The listing builds one solid part. Answer for the finished solid, in the listing's coordinates (mm). A direction names the side the tool comes from. Give positions to 0.01 mm unless a question says otherwise; leave off trailing zeros. Write each loop counter-clockwise with the first axis right and the second up, starting at its lowest first coordinate (ties: lowest second). Pieces come first, ordered by that corner, then holes. Notation, with made-up numbers: (-3.5, -10) - (6.5, -10) arc R25 ccw to (6.5, 19) - close; hole circle Ø5 at (65.5, -8). An arc over 180 degrees is marked (long way). One line per question, with ' | ' between items. Start each with the question number.
1. Find the intervals of material crossed by L1, parallel to Z at x = 0, y = -12; L2, parallel to Z at x = 8, y = 29.5; L3, parallel to X at y = -1, z = 33, in increasing order. Write a range as from..to.
2. The mould has two halves that part along Z. Classify faces 1 (the face through (24.77, -0.89, -58.47)), 2 (the face through (-1, -63.5, 1)), 3 (the face through (-59.728, -0.889, -21.558)), 4 (the face through (69.85, -0.89, -0.14)): +Z half, -Z half, draft (parallel to the pull), parting line (faces both ways), or undercut.
3. Given P1, Ø5, axis at y = 37.5, z = 25.5, coming from the -X side; P2, Ø2, axis at y = 20, z = -40, coming from the -X side; P3, Ø8, axis at x = -8.5, z = -7, coming from the +Y side, each flat-ended and moving along its own axis, determine where each tip first touches the part or whether it passes through.
4. A cutting plane is placed at A-A (y = -33). Determine the outline of the cut face in (x, z), then the cut area to 3 significant figures.
5. For faces 5 (the face through (50.57, 0.89, -48.17)), 6 (the face through (52.35, -0.89, -41.63)), 7 (the face through (53.17, -1, 43)), determine the directions among +Z, -Z, +X, -X, +Y, -Y from which every point of the face is accessible in a straight line to the end or side of a thin tool.
6. A cutting plane is placed at B-B (y = -14). Determine the outline of the cut face in (x, z), then the cut area to 3 significant figures.
```python
from build123d import *

# Parameters (mm, degrees)
F1_DEPTH = 63.5
F2_D     = 114.3
F2_DEPTH = 63.501
F3_D     = 114.3
F3_DEPTH = 25.4
F3_TIP   = 34.3391843774


with BuildPart() as f1:
    # F0 (on Front) → F1 (new body, symmetric)
    with BuildSketch(Plane.XZ):
        with BuildLine():
            ThreePointArc((63.1825, -6.3420575329), (63.4205753285, -3.175), (63.5, 0))
            ThreePointArc((63.5, 0), (63.4205753285, 3.175), (63.1825, 6.3420575329))
            ThreePointArc((63.1825, 6.3420575329), (57.15, 0), (63.1825, -6.3420575329))
        make_face()
        with BuildLine():
            ThreePointArc((63.1825, 6.3420575329), (63.4205753285, 3.175), (63.5, 0))
            ThreePointArc((63.5, 0), (63.4205753285, -3.175), (63.1825, -6.3420575329))
            ThreePointArc((63.1825, -6.3420575329), (67.8764354788, -4.6010121169), (69.85, 0))
            ThreePointArc((69.85, 0), (67.8764354788, 4.6010121169), (63.1825, 6.3420575329))
        make_face()
        with BuildLine():
            ThreePointArc((63.1825, -6.3420575329), (57.15, 0), (63.1825, 6.3420575329))
            ThreePointArc((63.1825, 6.3420575329), (59.2684226035, 22.7926321889), (51.1514073356, 37.6268989898))
            Line((51.1514073356, 37.6268989898), (44.3948691925, 35.4315666688))
            Line((44.3948691925, 35.4315666688), (38.9713217069, 42.8964393729))
            Line((38.9713217069, 42.8964393729), (42.2479521953, 47.4063343373))
            ThreePointArc((42.2479521953, 47.4063343373), (25.5434749418, 58.1358829631), (6.3420575329, 63.1825))
            ThreePointArc((6.3420575329, 63.1825), (0, 57.15), (-6.3420575329, 63.1825))
            ThreePointArc((-6.3420575329, 63.1825), (-26.2258003585, 57.831283883), (-43.351850487, 46.3989984736))
            Line((-43.351850487, 46.3989984736), (-40.1734631197, 40.6496002242))
            Line((-40.1734631197, 40.6496002242), (-46.4740063985, 33.9085063805))
            Line((-46.4740063985, 33.9085063805), (-51.9747429826, 36.4811744862))
            ThreePointArc((-51.9747429826, 36.4811744862), (-59.5179741382, 22.132798162), (-63.1825, 6.3420575329))
            ThreePointArc((-63.1825, 6.3420575329), (-58.8989878831, 4.3764354788), (-57.15, 0))
            ThreePointArc((-57.15, 0), (-58.8989878831, -4.3764354788), (-63.1825, -6.3420575329))
            ThreePointArc((-63.1825, -6.3420575329), (-59.6526265915, -21.7672722391), (-52.4184059941, -35.8407688679))
            Line((-52.4184059941, -35.8407688679), (-50.8226124015, -33.6443474184))
            Line((-50.8226124015, -33.6443474184), (-42.0471282301, -36.4956750697))
            Line((-42.0471282301, -36.4956750697), (-42.0471282301, -45.7227651753))
            Line((-42.0471282301, -45.7227651753), (-43.5515690674, -46.2115876352))
            ThreePointArc((-43.5515690674, -46.2115876352), (-26.3504546537, -57.7745925087), (-6.3420575329, -63.1825))
            ThreePointArc((-6.3420575329, -63.1825), (0, -57.15), (6.3420575329, -63.1825))
            ThreePointArc((6.3420575329, -63.1825), (25.0210307502, -58.3626423339), (41.3908210079, -48.1565149932))
            Line((41.3908210079, -48.1565149932), (39.1545134974, -46.9573614133))
            Line((39.1545134974, -46.9573614133), (40.7886670188, -37.876131646))
            Line((40.7886670188, -37.876131646), (49.9304109745, -36.6240496733))
            Line((49.9304109745, -36.6240496733), (50.7049691251, -38.2263797138))
            ThreePointArc((50.7049691251, -38.2263797138), (59.1332512734, -23.1410586153), (63.1825, -6.3420575329))
        make_face()
        with BuildLine():
            Line((44.3948691925, 35.4315666688), (51.1514073356, 37.6268989898))
            ThreePointArc((51.1514073356, 37.6268989898), (46.9549723579, 42.7490417539), (42.2479521953, 47.4063343373))
            Line((42.2479521953, 47.4063343373), (38.9713217069, 42.8964393729))
            Line((38.9713217069, 42.8964393729), (44.3948691925, 35.4315666688))
        make_face()
        with BuildLine():
            ThreePointArc((42.2479521953, 47.4063343373), (46.9549723579, 42.7490417539), (51.1514073356, 37.6268989898))
            Line((51.1514073356, 37.6268989898), (53.170353364, 38.28289432))
            Line((53.170353364, 38.28289432), (53.170353364, 47.5099844257))
            Line((53.170353364, 47.5099844257), (44.3948691925, 50.361312077))
            Line((44.3948691925, 50.361312077), (42.2479521953, 47.4063343373))
        make_face()
        with BuildLine():
            Line((53.9461659342, -44.9314502248), (50.7049691251, -38.2263797138))
            ThreePointArc((50.7049691251, -38.2263797138), (46.3147982477, -43.4417939694), (41.3908210079, -48.1565149932))
            Line((41.3908210079, -48.1565149932), (47.286295034, -51.3177880964))
            Line((47.286295034, -51.3177880964), (53.9461659342, -44.9314502248))
        make_face()
        with BuildLine():
            ThreePointArc((41.3908210079, -48.1565149932), (46.3147982477, -43.4417939694), (50.7049691251, -38.2263797138))
            Line((50.7049691251, -38.2263797138), (49.9304109745, -36.6240496733))
            Line((49.9304109745, -36.6240496733), (40.7886670188, -37.876131646))
            Line((40.7886670188, -37.876131646), (39.1545134974, -46.9573614133))
            Line((39.1545134974, -46.9573614133), (41.3908210079, -48.1565149932))
        make_face()
        with BuildLine():
            ThreePointArc((-6.3420575329, 63.1825), (0, 57.15), (6.3420575329, 63.1825))
            ThreePointArc((6.3420575329, 63.1825), (0, 63.5), (-6.3420575329, 63.1825))
        make_face()
        with BuildLine():
            ThreePointArc((-6.3420575329, 63.1825), (0, 63.5), (6.3420575329, 63.1825))
            ThreePointArc((6.3420575329, 63.1825), (6.3480140727, 63.3412003363), (6.35, 63.5))
            ThreePointArc((6.35, 63.5), (-0.1587996637, 69.8480140727), (-6.3420575329, 63.1825))
        make_face()
        with BuildLine():
            ThreePointArc((6.35, -63.5), (6.3480140727, -63.3412003363), (6.3420575329, -63.1825))
            ThreePointArc((6.3420575329, -63.1825), (0, -63.5), (-6.3420575329, -63.1825))
            ThreePointArc((-6.3420575329, -63.1825), (-0.1587996637, -69.8480140727), (6.35, -63.5))
        make_face()
        with BuildLine():
            ThreePointArc((-6.3420575329, -63.1825), (0, -63.5), (6.3420575329, -63.1825))
            ThreePointArc((6.3420575329, -63.1825), (0, -57.15), (-6.3420575329, -63.1825))
        make_face()
        with BuildLine():
            Line((-40.1734631197, 40.6496002242), (-43.351850487, 46.3989984736))
            ThreePointArc((-43.351850487, 46.3989984736), (-47.9205661881, 41.6637652668), (-51.9747429826, 36.4811744862))
            Line((-51.9747429826, 36.4811744862), (-46.4740063985, 33.9085063805))
            Line((-46.4740063985, 33.9085063805), (-40.1734631197, 40.6496002242))
        make_face()
        with BuildLine():
            ThreePointArc((-51.9747429826, 36.4811744862), (-47.9205661881, 41.6637652668), (-43.351850487, 46.3989984736))
            Line((-43.351850487, 46.3989984736), (-44.6376493999, 48.7248855241))
            Line((-44.6376493999, 48.7248855241), (-53.6972115319, 46.9745924645))
            Line((-53.6972115319, 46.9745924645), (-54.8321425725, 37.8175665635))
            Line((-54.8321425725, 37.8175665635), (-51.9747429826, 36.4811744862))
        make_face()
        with BuildLine():
            Line((-50.8226124015, -48.5740928266), (-43.5515690674, -46.2115876352))
            ThreePointArc((-43.5515690674, -46.2115876352), (-48.2643501852, -41.2650275802), (-52.4184059941, -35.8407688679))
            Line((-52.4184059941, -35.8407688679), (-56.2461598872, -41.1092201225))
            Line((-56.2461598872, -41.1092201225), (-50.8226124015, -48.5740928266))
        make_face()
        with BuildLine():
            ThreePointArc((-52.4184059941, -35.8407688679), (-48.2643501852, -41.2650275802), (-43.5515690674, -46.2115876352))
            Line((-43.5515690674, -46.2115876352), (-42.0471282301, -45.7227651753))
            Line((-42.0471282301, -45.7227651753), (-42.0471282301, -36.4956750697))
            Line((-42.0471282301, -36.4956750697), (-50.8226124015, -33.6443474184))
            Line((-50.8226124015, -33.6443474184), (-52.4184059941, -35.8407688679))
        make_face()
        with BuildLine():
            ThreePointArc((-57.15, 0), (-58.8989878831, 4.3764354788), (-63.1825, 6.3420575329))
            ThreePointArc((-63.1825, 6.3420575329), (-63.5, 0), (-63.1825, -6.3420575329))
            ThreePointArc((-63.1825, -6.3420575329), (-58.8989878831, -4.3764354788), (-57.15, 0))
        make_face()
        with BuildLine():
            ThreePointArc((-63.1825, -6.3420575329), (-63.5, 0), (-63.1825, 6.3420575329))
            ThreePointArc((-63.1825, 6.3420575329), (-69.85, 0), (-63.1825, -6.3420575329))
        make_face()
    extrude(amount=F1_DEPTH, both=True)

    # F2 (through all, one way)
    with BuildSketch(Plane.XZ):
        with Locations((0, 0)):
            Circle(F2_D / 2)
    extrude(amount=-F2_DEPTH, mode=Mode.SUBTRACT)

    # F3
    with Locations(Plane(origin=(0, 0, 0), x_dir=(1, 0, 0), z_dir=(0, 1, 0))):
        with Locations((0, 0)):
            Hole(F3_D / 2, depth=F3_DEPTH)
            with Locations((0, 0, -(F3_DEPTH + F3_TIP / 2))):  # 118° drill point
                Cone(0, F3_D / 2, F3_TIP, mode=Mode.SUBTRACT)


solid = f1.part
```
Determined:
1) L1: -69.85..-57.15, 57.15..69.85 | L2: -62.99..-56.59, 56.59..62.99 | L3: -54.25..-46.66, 46.66..54.25
2) face 1: -Z half | face 2: draft | face 3: undercut | face 4: parting line
3) P1: x = -59.19 | P2: x = -56.17 | P3: y = -50.72
4) outline: (-63.18, -6.34) arc R63.5 ccw to (-52.42, -35.84) - (-56.25, -41.11) - (-50.82, -48.57) - (-43.55, -46.21) arc R63.5 ccw to (-6.34, -63.18) arc R6.35 ccw (long way) to (6.34, -63.18) arc R63.5 ccw to (41.39, -48.16) - (47.29, -51.32) - (53.95, -44.93) - (50.7, -38.23) arc R63.5 ccw to (63.18, -6.34) arc R6.35 ccw (long way) to (63.18, 6.34) arc R63.5 ccw to (51.15, 37.63) - (53.17, 38.28) - (53.17, 47.51) - (44.39, 50.36) - (42.25, 47.41) arc R63.5 ccw to (6.34, 63.18) arc R6.35 ccw (long way) to (-6.34, 63.18) arc R63.5 ccw to (-43.35, 46.4) - (-44.64, 48.72) - (-53.7, 46.97) - (-54.83, 37.82) - (-51.97, 36.48) arc R63.5 ccw to (-63.18, 6.34) arc R6.35 ccw (long way) to start; hole circle Ø89 at (0, 0) | area: 7,000 mm2
5) face 5: -Z, +X, +Y, -Y | face 6: +X, +Y, -Y | face 7: +Z, +X, +Y, -Y
6) outline: (-63.18, -6.34) arc R63.5 ccw to (-52.42, -35.84) - (-56.25, -41.11) - (-50.82, -48.57) - (-43.55, -46.21) arc R63.5 ccw to (-6.34, -63.18) arc R6.35 ccw (long way) to (6.34, -63.18) arc R63.5 ccw to (41.39, -48.16) - (47.29, -51.32) - (53.95, -44.93) - (50.7, -38.23) arc R63.5 ccw to (63.18, -6.34) arc R6.35 ccw (long way) to (63.18, 6.34) arc R63.5 ccw to (51.15, 37.63) - (53.17, 38.28) - (53.17, 47.51) - (44.39, 50.36) - (42.25, 47.41) arc R63.5 ccw to (6.34, 63.18) arc R6.35 ccw (long way) to (-6.34, 63.18) arc R63.5 ccw to (-43.35, 46.4) - (-44.64, 48.72) - (-53.7, 46.97) - (-54.83, 37.82) - (-51.97, 36.48) arc R63.5 ccw to (-63.18, 6.34) arc R6.35 ccw (long way) to start; hole circle Ø114.3 at (0, 0) | area: 2,960 mm2
